```python
from build123d import *

# Parameters (mm, degrees)
SKETCH4_W               = 41
SKETCH4_H               = 45
SKETCH4_R               = 4.25
BOSS_EXTRUDE1_DEPTH     = 20
SKETCH6_W               = 9.8
SKETCH6_H               = 152.4
BOSS_EXTRUDE2_DEPTH     = 20
SKETCH7_R               = 5
BOSS_EXTRUDE3_DEPTH     = 9.8
SKETCH8_R               = 5
CUT_EXTRUDE2_DEPTH      = 15
SKETCH5_R               = 8.25
CUT_EXTRUDE1_DEPTH      = 65
BOSS_EXTRUDE4_DEPTH     = 20
CUT_EXTRUDE3_DEPTH      = 86
CUT_EXTRUDE3_DEPTH_BACK = 86
BOSS_EXTRUDE5_START     = -1.5
BOSS_EXTRUDE5_DEPTH     = 1.5
CUT_EXTRUDE4_DEPTH      = 13.5
SKETCH13_R              = 5
BOSS_EXTRUDE6_DEPTH     = 4
SKETCH14_R              = 4
CUT_EXTRUDE5_DEPTH      = 10
CUT_EXTRUDE6_DEPTH      = 15


with BuildPart() as part:
    # Sketch4 → Boss-Extrude1 (new body)
    with BuildSketch(Plane.XY):
        Rectangle(SKETCH4_W, SKETCH4_H)
        with Locations((-11.95, 14.95)):
            Circle(SKETCH4_R, mode=Mode.SUBTRACT)
        with Locations((11.95, 14.95)):
            Circle(SKETCH4_R, mode=Mode.SUBTRACT)
        with Locations((11.95, -14.95)):
            Circle(SKETCH4_R, mode=Mode.SUBTRACT)
        with Locations((-11.95, -14.95)):
            Circle(SKETCH4_R, mode=Mode.SUBTRACT)
    extrude(amount=BOSS_EXTRUDE1_DEPTH)

    # Sketch6 → Boss-Extrude2 (add)
    with BuildSketch(Plane(origin=(0, 0, 0), x_dir=(-1, 0, 0), z_dir=(0, 0, -1))):
        with Locations((25.4, 53.7)):
            Rectangle(SKETCH6_W, SKETCH6_H)
    extrude(amount=-BOSS_EXTRUDE2_DEPTH)

    # Sketch7 → Boss-Extrude3 (add)
    with BuildSketch(Plane(origin=(-20.5, 0, 0), x_dir=(0, 0, -1), z_dir=(1, 0, 0))):
        with Locations((-10, 114.9)):
            Circle(SKETCH7_R)
        with Locations((-10, 86.9)):
            Circle(SKETCH7_R)
        with BuildLine():
            Line((0, 76.2), (0.583845628, 77.176915135))
            ThreePointArc((0.583845628, 77.176915135), (1.639462026, 79.646010822), (2, 82.306982798))
            Line((2, 82.306982798), (2, 123.885290943))
            ThreePointArc((2, 123.885290943), (1.549421785, 126.853210006), (0.238291287, 129.553673135))
            Line((0.238291287, 129.553673135), (0, 129.9))
            Line((0, 129.9), (0, 76.2))
        make_face()
        with BuildLine():
            Line((-20, 76.2), (-20.583845628, 77.176915135))
            ThreePointArc((-20.583845628, 77.176915135), (-21.639462026, 79.646010822), (-22, 82.306982798))
            Line((-22, 82.306982798), (-22, 123.885290943))
            ThreePointArc((-22, 123.885290943), (-21.549421785, 126.853210006), (-20.238291287, 129.553673135))
            Line((-20.238291287, 129.553673135), (-20, 129.9))
            Line((-20, 129.9), (-20, 76.2))
        make_face()
    extrude(amount=-BOSS_EXTRUDE3_DEPTH)

    # Sketch8 → Cut-Extrude2 (cut)
    with BuildSketch(Plane(origin=(-20.5, 0, 0), x_dir=(0, 0, -1), z_dir=(1, 0, 0))):
        with Locations((-10, 86.9)):
            Circle(SKETCH8_R)
        with Locations((-10, 114.9)):
            Circle(SKETCH8_R)
    extrude(amount=-CUT_EXTRUDE2_DEPTH, mode=Mode.SUBTRACT)

    # Sketch5 → Cut-Extrude1 (cut)
    with BuildSketch(Plane(origin=(20.5, 0, 0), x_dir=(0, 0, -1), z_dir=(1, 0, 0))):
        with Locations((-0.5, 0)):
            Circle(SKETCH5_R)
    extrude(amount=-CUT_EXTRUDE1_DEPTH, mode=Mode.SUBTRACT)

    # Sketch9 → Boss-Extrude4 (add)
    with BuildSketch(Plane(origin=(0, 0, 0), x_dir=(-1, 0, 0), z_dir=(0, 0, -1))):
        with BuildLine():
            Line((-20.5, 22.5), (-20.5, 62.5))
            ThreePointArc((-20.5, 62.5), (-19.035533906, 66.035533906), (-15.5, 67.5))
            Line((-15.5, 67.5), (20.5, 67.5))
            Line((20.5, 67.5), (20.5, 22.5))
            Line((20.5, 22.5), (-20.5, 22.5))
        make_face()
    extrude(amount=-BOSS_EXTRUDE4_DEPTH)

    # Sketch10 → Cut-Extrude3 (cut, two sides: drawn at the far end of the back side and taken through both)
    with BuildSketch(Plane.XY.offset(-CUT_EXTRUDE3_DEPTH_BACK)):
        Polygon((-30.3, -22.5), (-26.3, -22.5), (-26.3, 157.593855938), (-61.075791469, 162.523409413), (-64.522830675, 37.584660103), align=None)
    extrude(amount=CUT_EXTRUDE3_DEPTH + CUT_EXTRUDE3_DEPTH_BACK, mode=Mode.SUBTRACT)

    # Sketch11 → Boss-Extrude5 (add)
    with BuildSketch(Plane.ZY.offset(26.3).offset(BOSS_EXTRUDE5_START)):
        with BuildLine():
            Line((0, -8.234834546), (0, 8.234834546))
            ThreePointArc((0, 8.234834546), (8.75, 0), (0, -8.234834546))
        make_face()
    extrude(amount=BOSS_EXTRUDE5_DEPTH)

    # Sketch12 → Cut-Extrude4 (cut)
    with BuildSketch(Plane(origin=(-20.5, 0, 0), x_dir=(0, 0, -1), z_dir=(1, 0, 0))):
        with BuildLine():
            Line((-22, 123.885290943), (-30.820305045, 123.885290943))
            Line((-30.820305045, 123.885290943), (-25.068984461, 136.818732695))
            Line((-25.068984461, 136.818732695), (-2.479535984, 134.912757399))
            Line((-2.479535984, 134.912757399), (8.997050859, 125.264275664))
            Line((8.997050859, 125.264275664), (2, 123.885290943))
            ThreePointArc((2, 123.885290943), (-10, 129.9), (-22, 123.885290943))
        make_face()
    extrude(amount=-CUT_EXTRUDE4_DEPTH, mode=Mode.SUBTRACT)

    # Sketch13 → Boss-Extrude6 (add)
    with BuildSketch(Plane.ZY.offset(26.3)):
        with BuildLine():
            Line((0, -22.5), (20, -22.5))
            Line((20, -22.5), (20, 76.2))
            Line((20, 76.2), (20.583845628, 77.176915135))
            ThreePointArc((20.583845628, 77.176915135), (21.639462026, 79.646010822), (22, 82.306982798))
            Line((22, 82.306982798), (22, 123.885290943))
            ThreePointArc((22, 123.885290943), (10, 129.9), (-2, 123.885290943))
            Line((-2, 123.885290943), (-2, 82.306982798))
            ThreePointArc((-2, 82.306982798), (-1.639462026, 79.646010822), (-0.583845628, 77.176915135))
            Line((-0.583845628, 77.176915135), (0, 76.2))
            Line((0, 76.2), (0, -22.5))
        make_face()
        with Locations(Location((10, 114.9, 0), (0, 0, 180))):
            Circle(SKETCH13_R, mode=Mode.SUBTRACT)
        with Locations(Location((10, 86.9, 0), (0, 0, 180))):
            Circle(SKETCH13_R, mode=Mode.SUBTRACT)
    extrude(amount=BOSS_EXTRUDE6_DEPTH)

    # Sketch14 → Cut-Extrude5 (cut)
    with BuildSketch(Plane.ZY.offset(30.3)):
        Circle(SKETCH14_R)
    extrude(amount=-CUT_EXTRUDE5_DEPTH, mode=Mode.SUBTRACT)

    # Sketch16 → Cut-Extrude6 (cut)
    with BuildSketch(Plane(origin=(0, 0, 0), x_dir=(-1, 0, 0), z_dir=(0, 0, -1))):
        with BuildLine():
            Line((-7.337559311, 35.883172827), (8.281826454, 54.105327978))
            ThreePointArc((8.281826454, 54.105327978), (8.734653676, 57.347267148), (5.97851601, 59.113315631))
            Line((5.97851601, 59.113315631), (-2.674541305, 59.113315631))
            ThreePointArc((-2.674541305, 59.113315631), (-9.745609117, 56.184383443), (-12.674541305, 49.113315631))
            Line((-12.674541305, 49.113315631), (-12.674541305, 37.857488931))
            ThreePointArc((-12.674541305, 37.857488931), (-10.693408521, 35.012260431), (-7.337559311, 35.883172827))
        make_face()
        with BuildLine():
            Line((4.245024065, 32.065048559), (11.254642469, 40.242729553))
            ThreePointArc((11.254642469, 40.242729553), (14.573244191, 41.103975455), (16.53238784, 38.290326924))
            Line((16.53238784, 38.290326924), (16.53238784, 30.11264593))
            ThreePointArc((16.53238784, 30.11264593), (15.653708183, 27.991325586), (13.53238784, 27.11264593))
            Line((13.53238784, 27.11264593), (6.522769436, 27.11264593))
            ThreePointArc((6.522769436, 27.11264593), (3.797222895, 28.859092558), (4.245024065, 32.065048559))
        make_face()
    extrude(amount=-CUT_EXTRUDE6_DEPTH, mode=Mode.SUBTRACT)


solid = part.part
```
Source: CAD feature listing. Evaluate the final solid. Frame: model axes, mm. A direction names the side the tool comes from. Round coordinates to 2 decimals unless told otherwise and drop trailing zeros. Order: outer loops, then holes, each group sorted by start corner. A loop starts at its lowest first (then second) coordinate and runs counter-clockwise, first axis right, second up. Notation, with made-up numbers: (-16.5, 24.5) -> (3.5, 24.5) arc R16 ccw to (3.5, 53.5) -> close; hole circle Ø10 at (33.5, 6.5). An arc over 180 degrees is marked (long way). Use CSV: the item, a comma, the result in double quotes.
(1) Pull-direction query (Y, two-part tool) for faces 4 (the face through (-28, 0, 4)), 5 (the face through (-30.3, 55, 10)), 6 (the face through (-2, 67.5, 10)); classes: +Y half, -Y half, draft (parallel to the pull), parting line (faces both ways), or undercut.
Report:
face 4,"undercut"
face 5,"draft"
face 6,"+Y half"
(2) First-contact query: pin 1 Ø10 at (x, z) = (15, 15) entering from +Y; pin 2 Ø5 at (x, y) = (13, 20) entering from +Z; pin 3 Ø15 at (x, y) = (6, -12) entering from -Z; pin 4 Ø7 at (x, y) = (11.95, -14.95) entering from +Z. Flat tips, straight axial feed; report the tip coordinate or a pass-through.
Report:
pin 1,"y = 67.5"
pin 2,"z = 20"
pin 3,"z = 0"
pin 4,"through"
(3) Section C-C on y = 14.95. Return the cut outline in (x, z).
Report:
outline,"(-30.3, 0) -> (-16.2, 0) -> (-16.2, 20) -> (-30.3, 20) -> close; (-7.7, 0) -> (7.7, 0) -> (7.7, 20) -> (-7.7, 20) -> close; (16.2, 0) -> (20.5, 0) -> (20.5, 20) -> (16.2, 20) -> close"
(4) Ray query, L1, parallel to Y at x = -12, z = 16; L2, parallel to X at y = 15, z = 8; L3, parallel to Y at x = -25, z = 9.75. Return the intervals inside material, ascending.
Report:
L1,"-22.5 to -19.2, -10.7 to 10.7, 19.2 to 67.5"
L2,"-30.3 to -16.2, -7.7 to 7.7, 16.2 to 20.5"
L3,"-22.5 to 81.91, 91.89 to 109.91, 119.89 to 129.9"
(5) Section A-A on y = 114.9. Return the cut outline in (x, z).
Report:
outline,"(-30.3, -2) -> (-20.5, -2) -> (-20.5, 5) -> (-30.3, 5) -> close; (-30.3, 15) -> (-20.5, 15) -> (-20.5, 22) -> (-30.3, 22) -> close"
(6) Access query for faces 1 (the face through (-24.8, 0.1, 4.4)), 2 (the face through (-7.701, 36.097, 7.395)), 3 (the face through (19.07, 66, 9.86)). Directions: +Z, -Z, +X, -X, +Y, -Y. A direction counts if a zero-diameter tool reaches every point of the face in a straight line with its end or side. Return the directions, or none.
Report:
face 1,"-Z, +X"
face 2,"-Z"
face 3,"+Z, -Z, +X, +Y"
(7) Section D-D on y = 93.5. Return the cut outline in (x, z).
Report:
outline,"(-30.3, -2) -> (-20.5, -2) -> (-20.5, 22) -> (-30.3, 22) -> close"
(8) Section B-B on z = 12.75. Count the separate pieces of the cut face and the enclosed holes in it, and give its area (3 significant figures).
Report:
separate pieces,"3"
enclosed holes,"6"
area,"4,320 mm^2"
